Read the model definition and answer for the solid it produces. Units are mm, in the model's axes. Face numbers are marked on the shaded views. Round coordinates to 2 decimals unless told otherwise and drop trailing zeros. Loops run counter-clockwise (first coordinate to the right, second up) from the corner with the lowest first, then second, coordinate; pieces in that order, holes last. Notation, with made-up numbers: (28, 29.5) -> (59, 29.5) arc R10 ccw to (59, 38.5) -> close; hole circle Ø9 at (76.5, -25.75). An arc over 180 degrees is marked (long way). Put each result on its own line as item: value.
from build123d import *

# Parameters (mm, degrees)
SKIZZE1_R                            = 5
AUFSATZ_LINEAR_AUSTRAGEN1_DEPTH      = 9.3
SCHNITT_LINEAR_AUSTRAGEN1_DEPTH      = 12.682893477
SCHNITT_LINEAR_AUSTRAGEN1_DEPTH_BACK = 12.682893477
SKIZZE2_R                            = 1.5
SCHNITT_LINEAR_START                 = -10
SKIZZE9_R                            = 0.5
SCHNITT_LINEAR_AUSTRAGEN2_DEPTH      = 10


with BuildPart() as part:
    # Skizze1 → Aufsatz-Linear austragen1 (new body)
    with BuildSketch(Plane.XY):
        Circle(SKIZZE1_R)
    extrude(amount=AUFSATZ_LINEAR_AUSTRAGEN1_DEPTH)

    # Skizze2 → Schnitt-Linear austragen1 (cut, two sides: drawn at the far end of the back side and taken through both)
    with BuildSketch(Plane.XY.offset(9.3).offset(-SCHNITT_LINEAR_AUSTRAGEN1_DEPTH_BACK)):
        Circle(SKIZZE2_R)
    extrude(amount=SCHNITT_LINEAR_AUSTRAGEN1_DEPTH + SCHNITT_LINEAR_AUSTRAGEN1_DEPTH_BACK, mode=Mode.SUBTRACT)

    # Skizze8 → Ø1.0 (1) Durchmesser Bohrung3 (revolve, cut)
    with BuildSketch(Plane(origin=(0, 0, 2), x_dir=(0, 0, -1), z_dir=(1, 0, 0))):
        Polygon((0, 0), (0, 4.30043031), (0.5, 4), (0.5, 0), align=None)
    revolve(axis=Axis((0, -6.35, 2), (0, 1, 0)), mode=Mode.SUBTRACT)

    # Skizze9 → Schnitt-Linear austragen2 (cut)
    with BuildSketch(Plane(origin=(0, 0, 0), x_dir=(1, 0, 0), z_dir=(0, 1, 0)).offset(SCHNITT_LINEAR_START)):
        with Locations(Location((0, -2, 0), (0, 0, 90))):
            Circle(SKIZZE9_R)
    extrude(amount=SCHNITT_LINEAR_AUSTRAGEN2_DEPTH, mode=Mode.SUBTRACT)


solid = part.part
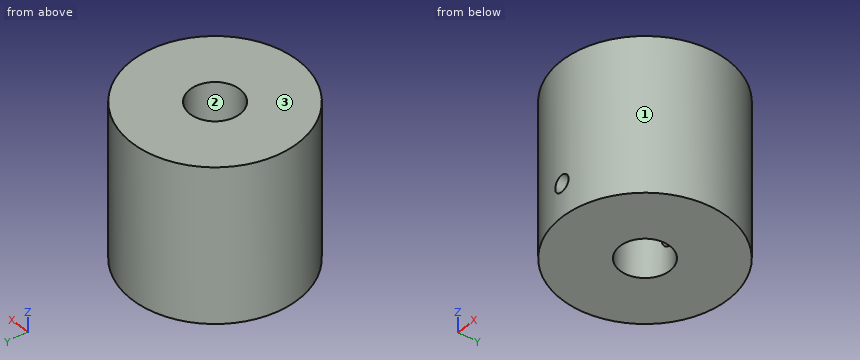
Item 1: The part is cut by section C-C (y = -2.75). Determine the outline of the cut face in (x, z).
Derived:
outline: (-4.18, 0) -> (4.18, 0) -> (4.18, 9.3) -> (-4.18, 9.3) -> close; hole circle Ø1 at (0, 2)
Item 2: The part is cut by section D-D (z = 5.5). Determine the outline of the cut face in (x, y), then the cut area to 3 significant figures.
Derived:
outline: circle Ø10 at (0, 0); hole circle Ø3 at (0, 0)
area: 71.5 mm^2
Item 3: The part is cut by section B-B (x = -1.25). Determine the outline of the cut face in (y, z).
Derived:
outline: (-4.84, 0) -> (-0.83, 0) -> (-0.83, 9.3) -> (-4.84, 9.3) -> close; (0.83, 0) -> (4.84, 0) -> (4.84, 9.3) -> (0.83, 9.3) -> close
Item 4: Find the intervals of material crossed by line 1 along Z through (x, y) = (0, 3.25); line 2 along Y through (x, z) = (0, 6.25); line 3 along Y through (x, z) = (-0.75, 0.5), in increasing order.
Derived:
line 1: z = 0 to 1.5, 2.5 to 9.3
line 2: y = -5 to -1.5, 1.5 to 5
line 3: y = -4.94 to -1.3, 1.3 to 4.94
Item 5: For a pull along X with two mould halves and no side action, classify the marked faces 1, 2 and 3 as pulls with the +X half, pulls with the -X half, needs draft (parallel to the pull), parting line crosses it, or undercut.
Derived:
face 1: parting line crosses it
face 2: undercut
face 3: needs draft
Item 6: The part is cut by section A-A (y = 0). Determine the outline of the cut face in (x, z).
Derived:
outline: (-5, 0) -> (-1.5, 0) -> (-1.5, 9.3) -> (-5, 9.3) -> close; (1.5, 0) -> (5, 0) -> (5, 9.3) -> (1.5, 9.3) -> close
Item 7: Flat-ended cylindrical pins translate along their axes: pin 1 Ø1 at (x, z) = (-4, 2.5) entering from -Y; pin 2 Ø3.5 at (x, y) = (0, 0) entering from +Z; pin 3 Ø3 at (y, z) = (3, 4) entering from +X. Find the tip coordinate at first contact, or state that the pin passes through.
Derived:
pin 1: stops at y = -3.57
pin 2: stops at z = 9.3
pin 3: stops at x = 4.77
